Answer from the drawing. Dimensions are ordinates in mm from the lowest x, y and z of the part. Round coordinates to 2 decimals unless told otherwise and drop trailing zeros. Loops run counter-clockwise (first coordinate to the right, second up) from the corner with the lowest first, then second, coordinate; pieces in that order, holes last. Notation, with made-up numbers: (37, 55) - (79, 55) arc R17 ccw to (79, 83) - close; hole circle Ø4 at (80.25, -33). An arc over 180 degrees is marked (long way). Answer as CSV lines item,"result". Start each with the question number.
Q1. Section A-A on x = 114.3 is taken. Count the separate pieces of the cut face and the enclosed holes in it, then the cut area to 3 significant figures.
Q2. Section C-C on z = 95.25 is taken. Write down the section's boundary in (x, y) (1 decimal).
Q3. Each of these flat-tipped pins is pushed along its axis until it touches: pin 1 Ø6.5 at (x, z) = (50.8, 88.9) entering from +Y (3 decimals); pin 2 Ø1.5 at (x, y) = (17.5, 0.5) entering from -Z (1 decimal); pin 3 Ø2.5 at (x, z) = (63.5, 82.55) entering from +Y. Where does it stop, or does it pass through?
Q4. Section B-B on x = 69.85 is taken. Write down the section's boundary in (y, z) (1 decimal), then the cut area to 3 significant figures.
Q5. Straight lines are drawn through the part: L1, parallel to X at y = 2.1, z = 82.55; L2, parallel to X at y = 2.15, z = 88.9; L3, parallel to Z at x = 58, y = 2.5. For each, find the intervals that lie inside material, in ascending order. Write a range as [from, to].
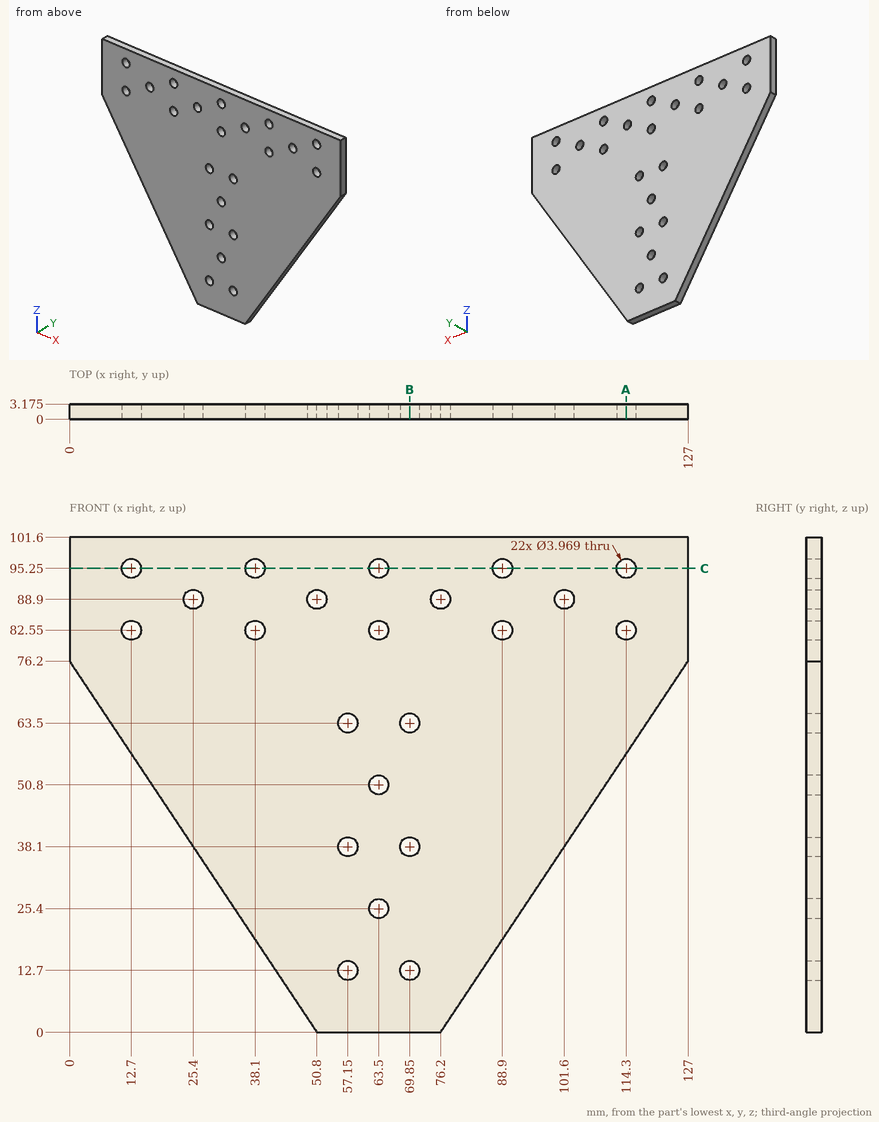
Findings:
1,separate pieces,"3"
1,enclosed holes,"0"
1,area,"116 mm^2"
2,outline,"(0, 0) - (10.7, 0) - (10.7, 3.2) - (0, 3.2) - close; (14.7, 0) - (36.1, 0) - (36.1, 3.2) - (14.7, 3.2) - close; (40.1, 0) - (61.5, 0) - (61.5, 3.2) - (40.1, 3.2) - close; (65.5, 0) - (86.9, 0) - (86.9, 3.2) - (65.5, 3.2) - close; (90.9, 0) - (112.3, 0) - (112.3, 3.2) - (90.9, 3.2) - close; (116.3, 0) - (127, 0) - (127, 3.2) - (116.3, 3.2) - close"
3,pin 1,"stops at y = 3.175"
3,pin 2,"stops at z = 48.8"
3,pin 3,"passes through"
4,outline,"(0, 0) - (3.2, 0) - (3.2, 10.7) - (0, 10.7) - close; (0, 14.7) - (3.2, 14.7) - (3.2, 36.1) - (0, 36.1) - close; (0, 40.1) - (3.2, 40.1) - (3.2, 61.5) - (0, 61.5) - close; (0, 65.5) - (3.2, 65.5) - (3.2, 101.6) - (0, 101.6) - close"
4,area,"285 mm^2"
5,L1,"x = [0, 10.72], [14.68, 36.12], [40.08, 61.52], [65.48, 86.92], [90.88, 112.32], [116.28, 127]"
5,L2,"x = [0, 23.42], [27.38, 48.82], [52.78, 74.22], [78.18, 99.62], [103.58, 127]"
5,L3,"z = [0, 10.91], [14.49, 36.31], [39.89, 61.71], [65.29, 101.6]"
